from build123d import *

# Parameters (mm, degrees)
PAD001_DEPTH         = 40
POCKET_DEPTH         = 101.001
PAD002_DEPTH         = 91.5
POCKET001_DEPTH      = 64
POCKET001_DEPTH_BACK = 64


with BuildPart() as part:
    # Sketch003 (on Sketch) → Pad001 (new body)
    with BuildSketch(Plane.XY):
        with BuildLine():
            Line((-20, -93.3), (20, -93.3))
            ThreePointArc((20, -93.3), (40.506097, -84.806097), (49, -64.3))
            Line((49, -64.3), (49, 64.3))
            ThreePointArc((49, 64.3), (40.506097, 84.806097), (20, 93.3))
            Line((20, 93.3), (-20, 93.3))
            ThreePointArc((-20, 93.3), (-40.506097, 84.806097), (-49, 64.3))
            Line((-49, 64.3), (-49, -64.3))
            ThreePointArc((-49, -64.3), (-40.506097, -84.806097), (-20, -93.3))
        make_face()
        with BuildLine():
            Line((-20, 90), (20, 90))
            ThreePointArc((45.7, 64.3), (38.172644, 82.472644), (20, 90))
            Line((45.7, 64.3), (45.7, -64.3))
            ThreePointArc((20, -90), (38.172644, -82.472644), (45.7, -64.3))
            Line((20, -90), (-20, -90))
            ThreePointArc((-45.7, -64.299999), (-38.172644, -82.472644), (-20, -90))
            Line((-45.7, -64.299999), (-45.7, 64.3))
            ThreePointArc((-20, 90), (-38.172644, 82.472644), (-45.7, 64.3))
        make_face(mode=Mode.SUBTRACT)
    extrude(amount=PAD001_DEPTH)

    # Sketch004 (on Face7 of Pad001) → Pocket (cut, through all)
    with BuildSketch(Plane(origin=(-52, 0, 0), x_dir=(0, -1, 0), z_dir=(-1, 0, 0))):
        with BuildLine():
            Line((-48.5, 40), (-59.133539, 40))
            Line((-59.133539, 40), (-64.3, 25.805264))
            Line((-64.3, 25.805264), (-99.376816, 25.805264))
            Line((-99.376816, 25.805264), (-99.376816, 55.805264))
            Line((-99.376816, 55.805264), (102.829521, 55.805264))
            Line((102.829521, 55.805264), (102.829521, 25.805264))
            Line((102.829521, 25.805264), (64.3, 25.805264))
            Line((64.3, 25.805264), (59.133539, 40))
            Line((59.133539, 40), (48.5, 40))
            ThreePointArc((40.1, 40), (44.3, 35.8), (48.5, 40))
            Line((28.1, 40), (40.1, 40))
            Line((22.933539, 25.805264), (28.1, 40))
            Line((-22.933539, 25.805264), (22.933539, 25.805264))
            Line((-28.1, 40), (-22.933539, 25.805264))
            Line((-40.1, 40), (-28.1, 40))
            ThreePointArc((-48.5, 40), (-44.3, 35.8), (-40.1, 40))
        make_face()
    extrude(amount=-POCKET_DEPTH, mode=Mode.SUBTRACT)

    # Sketch005 (on Face15 of Pocket) → Pad002 (join)
    with BuildSketch(Plane(origin=(45.7, 0, 0), x_dir=(0, -1, 0), z_dir=(-1, 0, 0))):
        with BuildLine():
            Line((-60.5, 40), (-63.300706, 0))
            Line((-63.300706, 0), (-60.300706, 0))
            Line((-60.300706, 0), (-58.565336, 24.784757))
            Line((-58.565336, 24.784757), (-29.090411, 24.784757))
            Line((-29.090411, 24.784757), (-25.816907, 0))
            Line((-25.816907, 0), (-22.816907, 0))
            Line((-22.816907, 0), (-28.1, 40))
            Line((-33.1, 40), (-28.1, 40))
            ThreePointArc((-55.5, 40), (-44.3, 28.8), (-33.1, 40))
            Line((-60.5, 40), (-55.5, 40))
        make_face()
        with BuildLine():
            Line((28.1, 40), (22.816907, 0))
            Line((25.816907, 0), (22.816907, 0))
            Line((29.090411, 24.784757), (25.816907, 0))
            Line((29.090411, 24.784757), (58.565336, 24.784757))
            Line((58.565336, 24.784757), (60.300706, 0))
            Line((60.300706, 0), (63.300706, 0))
            Line((63.300706, 0), (60.5, 40))
            Line((55.5, 40), (60.5, 40))
            ThreePointArc((33.1, 40), (44.3, 28.8), (55.5, 40))
            Line((28.1, 40), (33.1, 40))
        make_face()
    extrude(amount=PAD002_DEPTH)

    # Sketch006 → Pocket001 (cut, two sides)
    with BuildSketch(Plane.XZ) as pocket001_sk:
        Polygon((-39.8, 40), (-39.8, 29), (-45.7, 0), (45.7, 0), (39.8, 29), (39.8, 40), align=None)
    extrude(amount=-POCKET001_DEPTH, mode=Mode.SUBTRACT)
    extrude(pocket001_sk.sketch, amount=POCKET001_DEPTH_BACK, mode=Mode.SUBTRACT)


solid = part.part
The model under review builds one solid part; all positions refer to its coordinate system, in mm. A direction names the side the tool comes from. Give positions to 0.01 mm unless a question says otherwise; leave off trailing zeros. Order: outer loops, then holes, each group sorted by start corner. A loop starts at its lowest first (then second) coordinate and runs counter-clockwise, first axis right, second up. Notation, with made-up numbers: (20.5, 88.5) -> (69.5, 88.5) arc R33 cw to (69.5, 124.5) -> close; hole circle Ø1 at (33.25, 51.5). An arc over 180 degrees is marked (long way). Write item = value, one per line. Start each with the question number.
(1) Tool access review of faces 4 (the flat face through (-43, 44, 24.785)), 5 (the flat face through (39.8, -57, 33)), 6 (the cylindrical face through (37.972, -82.671, 12.722)), 7 (the flat face through (45.7, -44, 34)): name each direction out of +Z, -Z, +X, -X, +Y, -Y from which nothing blocks a thin tool from reaching the whole face with its end or side.
(2) Take a section at C-C (z = 33). State how many separate pieces and enclosed holes the cut face has, plus the area to 3 significant figures.
(3) For pin 1 Ø2.5 at (x, y) = (-43, -37.5) entering from -Z; pin 2 Ø4 at (x, z) = (38, 31) entering from +Y; pin 3 Ø8 at (x, z) = (9, 30) entering from -Y; pin 4 Ø3 at (y, z) = (70.5, 24) entering from +X, all flat-tipped, find the tip position at first contact; note any pin that passes through.
(4) Take a section at B-B (y = 19). Write out the cut boundary in (x, z).
(5) For L1, parallel to X at y = 54, z = 2; L2, parallel to X at y = -58, z = 33; L3, parallel to Y at x = 35, z = 5, list the stretches that pass through material, from the lowest coordinate up. Write a range as from..to.
(6) Take a section at A-A (x = -7.5). Write out the cut boundary in (y, z).
(7) Take a section at D-D (y = 44.3). Write out the cut boundary in (x, z), plus the area to 3 significant figures.
(8) Draft analysis for pull direction X (two halves, no side actions). For faces 1 (the cylindrical face through (-40.73, -84.58, 12.72)), 2 (the flat face through (-47, 0, 25.805)), 3 (the flat face through (40.58, -42.96, 25.17)), state which applies: +X half, -X half, draft (parallel to the pull), parting line (faces both ways), or undercut.
Returned:
q1.face_4 = -Z
q1.face_5 = +Z, -Z, +Y, -Y
q1.face_6 = +Z, -Z
q1.face_7 = +Z
q2.separate_pieces = 4
q2.enclosed_holes = 0
q2.area = 862 mm²
q3.pin_1 = 24.78
q3.pin_2 = 61.19
q3.pin_3 = through
q3.pin_4 = 48.62
q4.outline = (-49, 0) -> (-45.7, 0) -> (-45.7, 25.81) -> (-49, 25.81) -> close; (45.7, 0) -> (49, 0) -> (49, 25.81) -> (45.7, 25.81) -> close
q5.L1 = -49..-45.7, 45.7..49
q5.L2 = -49..-39.8, 39.8..49
q5.L3 = -89.12..-85.17, 85.17..89.12
q6.outline = (-93.3, 0) -> (-90, 0) -> (-90, 25.81) -> (-93.3, 25.81) -> close; (90, 0) -> (93.3, 0) -> (93.3, 25.81) -> (90, 25.81) -> close
q7.outline = (-49, 0) -> (-45.7, 0) -> (-45.7, 24.78) -> (-40.66, 24.78) -> (-39.84, 28.8) -> (-45.7, 28.8) -> (-45.7, 35.8) -> (-49, 35.8) -> close; (39.84, 28.8) -> (40.66, 24.78) -> (45.7, 24.78) -> (45.7, 0) -> (49, 0) -> (49, 35.8) -> (45.7, 35.8) -> (45.7, 28.8) -> close
q7.area = 280 mm²
q8.face_1 = -X half
q8.face_2 = draft
q8.face_3 = undercut
